Verification items for the finished model (mm, model axes). Face numbers are marked on the shaded views. A direction names the side the tool comes from. Coordinates: 2 decimals unless noted, no trailing zeros. Order: outer loops, then holes, each group sorted by start corner. A loop starts at its lowest first (then second) coordinate and runs counter-clockwise, first axis right, second up. Notation, with made-up numbers: M -38.5,16.25 L -1.5,16.25 A36 cw -1.5,51.25 Z; hole C 57,2 d5. An arc over 180 degrees is marked long. Return JSON: item names as keys, results as strings. Group by question number.
1. Gauge pin test, flat end, axial feed: pin 1 (4.5 mm diameter, centred on x = 18, y = -5.5, fed in from +Z). Record the tip position at first contact, or that the pin passes through.
2. Section check C-C, the plane x = -40. Record the cut outline in (y, z).
3. Set-up check for the marked faces 1 and 2: record each of +Z, -Z, +X, -X, +Y, -Y from which the full face is reachable in a straight line by a thin tool's end or side.
4. Section check D-D, the plane z = 11. Record the cut outline in (x, y).
5. Material ranges on line 1 along X through (y, z) = (-6, 1.9); line 2 along Y through (x, z) = (50, 0.7); line 3 along Z through (x, y) = (40, -0.55), recorded low to high.
6. Section check A-A, the plane y = -6. Record the cut outline in (x, z).
7. Section check B-B, the plane z = 6. Record the cut outline in (x, y).
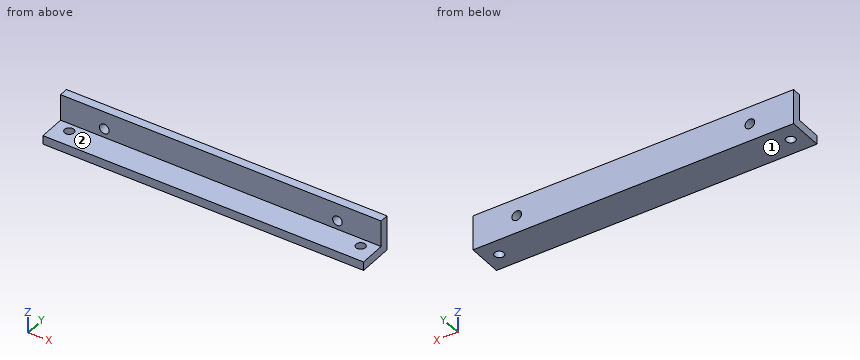
```python
from build123d import *

# Parameters (mm, degrees)
F1_DEPTH = 55
F3_D     = 3.2
F5_D     = 3.3


with BuildPart() as f1:
    # F0 (on Right) → F1 (new body, symmetric)
    with BuildSketch(Plane.YZ):
        Polygon((-12, 0), (0, 0), (0, 12), (-3, 12), (-3, 3), (-12, 3), align=None)
    extrude(amount=F1_DEPTH, both=True)

    # F3 (through all)
    with Locations(Plane(origin=(0, 0, 0), x_dir=(1, 0, 0), z_dir=(0, 0, -1))):
        with Locations((-50, 6), (50, 6)):
            Hole(F3_D / 2)

    # F5 (through all)
    with Locations(Plane(origin=(0, 0, 0), x_dir=(-1, 0, 0), z_dir=(0, 1, 0))):
        with Locations((40, 6), (-40, 6)):
            Hole(F5_D / 2)


solid = f1.part
```
Answers follow:
{
 "1": {"pin 1": "z = 3"},
 "2": {"outline": "M -12,0 L 0,0 L 0,4.35 L -3,4.35 L -3,3 L -12,3 Z; M -3,7.65 L 0,7.65 L 0,12 L -3,12 Z"},
 "3": {"face 1": "-Z, +X, -X, +Y, -Y", "face 2": "+Z, +X, -X, -Y"},
 "4": {"outline": "M -55,-3 L 55,-3 L 55,0 L -55,0 Z"},
 "5": {"line 1": "-55 to -51.6, -48.4 to 48.4, 51.6 to 55", "line 2": "-12 to -7.6, -4.4 to 0", "line 3": "0 to 4.35, 7.65 to 12"},
 "6": {"outline": "M -55,0 L -51.6,0 L -51.6,3 L -55,3 Z; M -48.4,0 L 48.4,0 L 48.4,3 L -48.4,3 Z; M 51.6,0 L 55,0 L 55,3 L 51.6,3 Z"},
 "7": {"outline": "M -55,-3 L -41.65,-3 L -41.65,0 L -55,0 Z; M -38.35,-3 L 38.35,-3 L 38.35,0 L -38.35,0 Z; M 41.65,-3 L 55,-3 L 55,0 L 41.65,0 Z"}
}
